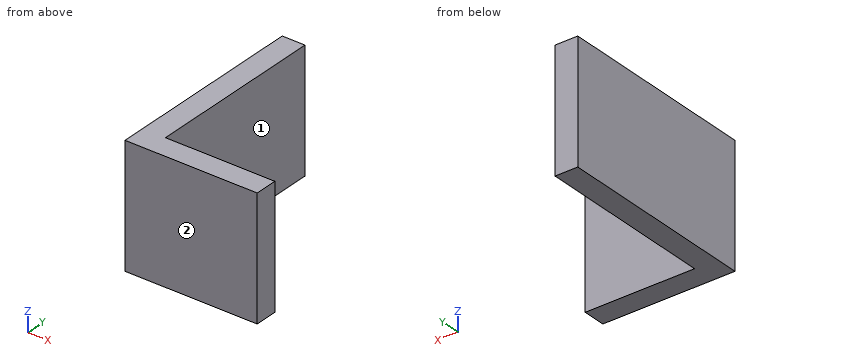
Autodesk Inventor part; units mm, degrees
ref_plane "YZ Plane" through (0, 0, 0) normal (1, 0, 0) x (0, 1, 0)
ref_plane "XZ Plane" through (0, 0, 0) normal (0, 1, 0) x (-1, 0, 0)
ref_plane "XY Plane" through (0, 0, 0) normal (0, 0, 1) x (1, 0, 0)
sketch "Boceto3" plane through (0, 0, 0) normal (0, 0, 1) x (1, 0, 0)
  line L0 (-681.5559, 400.996) -> (-581.5559, 400.996)
  line L1 (-101.5559, -489.004) -> (-681.5559, -489.004)
  line L2 (-681.5559, -489.004) -> (-681.5559, 400.996)
  line L3 (-101.5559, -489.004) -> (-101.5559, -389.004)
  line L4 (-101.5559, -389.004) -> (-581.5559, -389.004)
  line L5 (-581.5559, -389.004) -> (-581.5559, 400.996)
  point P0 (0, 0)
  dimension "d0" = 580
  dimension "d2" = 100
  dimension "d3" = 480
extrude "Extrusión1" add sketch "Boceto3" along normal blind 530
properties part number "silla aleta" material "Sillas"
Input: part model. Units: mm. Frame: model coordinates. Face numbers are marked on the shaded views. A direction names the side the tool comes from. Give positions to 0.01 mm unless a question says otherwise; leave off trailing zeros. Order: outer loops, then holes, each group sorted by start corner. A loop starts at its lowest first (then second) coordinate and runs counter-clockwise, first axis right, second up. Notation, with made-up numbers: M 31.5,58.25 L 76.5,58.25 A17 ccw 76.5,87.25 Z; hole C -11.5,-19 d2. An arc over 180 degrees is marked long. Answer as a JSON object with one key per item and string values.
1. Cut plane A-A, the plane z = 152.5. Output: boundary loops of the cut face in (x, y), and give its area (3 significant figures).
Result sheet:
{"outline": "M -681.56,-489 L -101.56,-489 L -101.56,-389 L -581.56,-389 L -581.56,401 L -681.56,401 Z", "area": "137,000 mm²"}
2. First-contact query: P1, Ø2, axis at y = -373, z = 161.5, coming from the +X side. Flat tip, straight axial feed; report the tip coordinate or a pass-through.
Result sheet:
{"P1": "x = -581.56"}
3. Ray query, line 1 (X direction, y = 7, z = 274); line 2 (Y direction, x = -548, z = 297.5). Return the intervals inside material, ascending. Write a range as [from, to].
Result sheet:
{"line 1": "[-681.56, -581.56]", "line 2": "[-489, -389]"}
4. Cut plane C-C, the plane x = -441. Output: boundary loops of the cut face in (y, z), and give its area (3 significant figures).
Result sheet:
{"outline": "M -489,0 L -389,0 L -389,530 L -489,530 Z", "area": "53,000 mm²"}
5. Cut plane B-B, the plane y = -71.5. Output: boundary loops of the cut face in (x, z), and give its area (3 significant figures).
Result sheet:
{"outline": "M -681.56,0 L -581.56,0 L -581.56,530 L -681.56,530 Z", "area": "53,000 mm²"}
6. Reachability of the marked faces 1 and 2 from +Z, -Z, +X, -X, +Y, -Y: full face, straight path, thin tool, end or side. Return the list, or none.
Result sheet:
{"face 1": "+Z, -Z, +X, +Y", "face 2": "+Z, -Z, +X, -X, -Y"}
